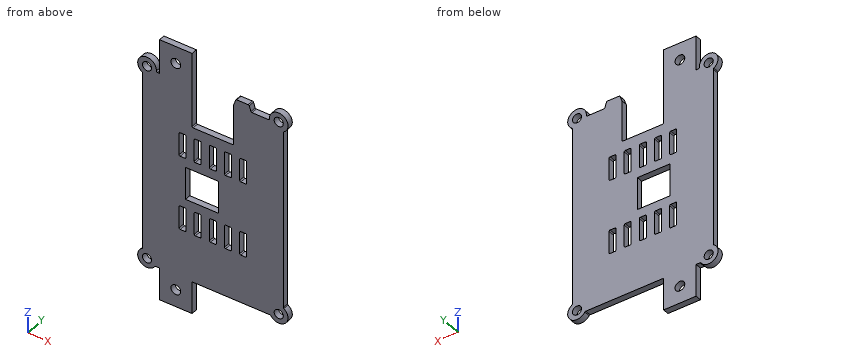
from build123d import *

# Parameters (mm, degrees)
BASEPLATE_OUTLINE_R = 2.1
BASEPLATE_DEPTH     = 2.8
CUT_EXTRUDE1_REACH  = 115.438
SKETCH3_W           = 19.2
SKETCH3_H           = 19.147905432
SKETCH3_W_2         = 15.1
SKETCH3_H_2         = 15.1
SKETCH3_W_3         = 3.2
SKETCH3_H_3         = 11.1
FILLET1_R           = 0.5
SKETCH4_W           = 15
SKETCH4_H           = 35
SKETCH4_R           = 2.25
SKETCH4_H_2         = 15
BOSS_EXTRUDE1_DEPTH = 2.8


# Read off the part's stored shape, not the designer's step: BasePlate
with BuildPart() as part:
    # BasePlate outline → BasePlate (new body)
    with BuildSketch(Plane(origin=(0, 0, 0), x_dir=(1, 0, 0), z_dir=(0, 1, 0))):
        with BuildLine():
            Line((43.502626614, -5.852332608), (48.792614178, -5.852332608))
            ThreePointArc((48.792614178, -5.852332608), (49.082078508, -5.760021707), (49.264659986, -5.517174213))
            Line((49.264659986, -5.517174213), (50.078201202, -3.187491002))
            ThreePointArc((50.078201202, -3.187491002), (50.26078268, -2.944643509), (50.55024701, -2.852332608))
            Line((50.55024701, -2.852332608), (58.116695703, -2.852332608))
            ThreePointArc((58.116695703, -2.852332608), (58.484685739, -3.013831008), (58.614956567, -3.393999275))
            ThreePointArc((58.614956567, -3.393999275), (64.799237397, -7.61016844), (65.229166667, -0.137781095))
            ThreePointArc((65.229166667, -0.137781095), (65.061014427, 0.043158816), (65, 0.282515593))
            Line((65, 0.282515593), (65, 83.012819192))
            ThreePointArc((65, 83.012819192), (65.061014427, 83.252175969), (65.229166667, 83.433115879))
            ThreePointArc((65.229166667, 83.433115879), (65.940559159, 90.088226551), (59.285448487, 89.376834059))
            ThreePointArc((59.285448487, 89.376834059), (59.104508577, 89.208681819), (58.8651518, 89.147667392))
            Line((58.8651518, 89.147667392), (6.1348482, 89.147667392))
            ThreePointArc((6.1348482, 89.147667392), (5.895491423, 89.208681819), (5.714551513, 89.376834059))
            ThreePointArc((5.714551513, 89.376834059), (-0.940559159, 90.088226551), (-0.229166667, 83.433115879))
            ThreePointArc((-0.229166667, 83.433115879), (-0.061014427, 83.252175969), (0, 83.012819192))
            Line((0, 83.012819192), (0, 0.282515593))
            ThreePointArc((0, 0.282515593), (-0.061014427, 0.043158816), (-0.229166667, -0.137781095))
            ThreePointArc((-0.229166667, -0.137781095), (0.200762603, -7.61016844), (6.385043433, -3.393999275))
            ThreePointArc((6.385043433, -3.393999275), (6.515314261, -3.013831008), (6.883304297, -2.852332608))
            Line((6.883304297, -2.852332608), (14.44975299, -2.852332608))
            ThreePointArc((14.44975299, -2.852332608), (14.73921732, -2.944643509), (14.921798798, -3.187491002))
            Line((14.921798798, -3.187491002), (15.735340014, -5.517174213))
            ThreePointArc((15.735340014, -5.517174213), (15.917921492, -5.760021707), (16.207385822, -5.852332608))
            Line((16.207385822, -5.852332608), (21.497373386, -5.852332608))
            ThreePointArc((21.497373386, -5.852332608), (21.786837716, -5.760021707), (21.969419194, -5.517174213))
            Line((21.969419194, -5.517174213), (22.78296041, -3.187491002))
            ThreePointArc((22.78296041, -3.187491002), (22.965541888, -2.944643509), (23.255006218, -2.852332608))
            Line((23.255006218, -2.852332608), (41.744993782, -2.852332608))
            ThreePointArc((41.744993782, -2.852332608), (42.034458112, -2.944643509), (42.21703959, -3.187491002))
            Line((42.21703959, -3.187491002), (43.030580806, -5.517174213))
            ThreePointArc((43.030580806, -5.517174213), (43.213162284, -5.760021707), (43.502626614, -5.852332608))
        make_face()
        with Locations((2.1, -3.752332608)):
            Circle(BASEPLATE_OUTLINE_R, mode=Mode.SUBTRACT)
        with Locations((62.9, -3.752332608)):
            Circle(BASEPLATE_OUTLINE_R, mode=Mode.SUBTRACT)
        with Locations((2.1, 87.047667392)):
            Circle(BASEPLATE_OUTLINE_R, mode=Mode.SUBTRACT)
        with Locations((62.9, 87.047667392)):
            Circle(BASEPLATE_OUTLINE_R, mode=Mode.SUBTRACT)
    extrude(amount=BASEPLATE_DEPTH)

    # Sketch3 → Cut-Extrude1 (cut, up to next)
    with BuildSketch(Plane(origin=(0, 2.8, 0), x_dir=(1, 0, 0), z_dir=(0, 1, 0)), mode=Mode.PRIVATE) as cut_extrude1_sk1:
        with Locations((32.5, 6.573714676)):
            Rectangle(SKETCH3_W, SKETCH3_H)
    cut_extrude1_tool1 = extrude(cut_extrude1_sk1.sketch, amount=-CUT_EXTRUDE1_REACH, mode=Mode.PRIVATE) & part.part
    # Sketch3 → Cut-Extrude1 (cut, up to next)
    with BuildSketch(Plane(origin=(0, 2.8, 0), x_dir=(1, 0, 0), z_dir=(0, 1, 0)), mode=Mode.PRIVATE) as cut_extrude1_sk2:
        with Locations((27.45, 43.897667392)):
            Rectangle(SKETCH3_W_2, SKETCH3_H_2)
    cut_extrude1_tool2 = extrude(cut_extrude1_sk2.sketch, amount=-CUT_EXTRUDE1_REACH, mode=Mode.PRIVATE) & part.part
    # Sketch3 → Cut-Extrude1 (cut, up to next)
    with BuildSketch(Plane(origin=(0, 2.8, 0), x_dir=(1, 0, 0), z_dir=(0, 1, 0)), mode=Mode.PRIVATE) as cut_extrude1_sk3:
        with Locations((32.5, 26.597667392)):
            Rectangle(SKETCH3_W_3, SKETCH3_H_3)
    cut_extrude1_tool3 = extrude(cut_extrude1_sk3.sketch, amount=-CUT_EXTRUDE1_REACH, mode=Mode.PRIVATE) & part.part
    # Sketch3 → Cut-Extrude1 (cut, up to next)
    with BuildSketch(Plane(origin=(0, 2.8, 0), x_dir=(1, 0, 0), z_dir=(0, 1, 0)), mode=Mode.PRIVATE) as cut_extrude1_sk4:
        with Locations((18.5, 26.597667392)):
            Rectangle(SKETCH3_W_3, SKETCH3_H_3)
    cut_extrude1_tool4 = extrude(cut_extrude1_sk4.sketch, amount=-CUT_EXTRUDE1_REACH, mode=Mode.PRIVATE) & part.part
    # Sketch3 → Cut-Extrude1 (cut, up to next)
    with BuildSketch(Plane(origin=(0, 2.8, 0), x_dir=(1, 0, 0), z_dir=(0, 1, 0)), mode=Mode.PRIVATE) as cut_extrude1_sk5:
        with Locations((39.5, 26.597667392)):
            Rectangle(SKETCH3_W_3, SKETCH3_H_3)
    cut_extrude1_tool5 = extrude(cut_extrude1_sk5.sketch, amount=-CUT_EXTRUDE1_REACH, mode=Mode.PRIVATE) & part.part
    # Sketch3 → Cut-Extrude1 (cut, up to next)
    with BuildSketch(Plane(origin=(0, 2.8, 0), x_dir=(1, 0, 0), z_dir=(0, 1, 0)), mode=Mode.PRIVATE) as cut_extrude1_sk6:
        with Locations((46.5, 26.597667392)):
            Rectangle(SKETCH3_W_3, SKETCH3_H_3)
    cut_extrude1_tool6 = extrude(cut_extrude1_sk6.sketch, amount=-CUT_EXTRUDE1_REACH, mode=Mode.PRIVATE) & part.part
    # Sketch3 → Cut-Extrude1 (cut, up to next)
    with BuildSketch(Plane(origin=(0, 2.8, 0), x_dir=(1, 0, 0), z_dir=(0, 1, 0)), mode=Mode.PRIVATE) as cut_extrude1_sk7:
        with Locations((25.5, 26.597667392)):
            Rectangle(SKETCH3_W_3, SKETCH3_H_3)
    cut_extrude1_tool7 = extrude(cut_extrude1_sk7.sketch, amount=-CUT_EXTRUDE1_REACH, mode=Mode.PRIVATE) & part.part
    # Sketch3 → Cut-Extrude1 (cut, up to next)
    with BuildSketch(Plane(origin=(0, 2.8, 0), x_dir=(1, 0, 0), z_dir=(0, 1, 0)), mode=Mode.PRIVATE) as cut_extrude1_sk8:
        with Locations((18.5, 61.197667392)):
            Rectangle(SKETCH3_W_3, SKETCH3_H_3)
    cut_extrude1_tool8 = extrude(cut_extrude1_sk8.sketch, amount=-CUT_EXTRUDE1_REACH, mode=Mode.PRIVATE) & part.part
    # Sketch3 → Cut-Extrude1 (cut, up to next)
    with BuildSketch(Plane(origin=(0, 2.8, 0), x_dir=(1, 0, 0), z_dir=(0, 1, 0)), mode=Mode.PRIVATE) as cut_extrude1_sk9:
        with Locations((32.5, 61.197667392)):
            Rectangle(SKETCH3_W_3, SKETCH3_H_3)
    cut_extrude1_tool9 = extrude(cut_extrude1_sk9.sketch, amount=-CUT_EXTRUDE1_REACH, mode=Mode.PRIVATE) & part.part
    # Sketch3 → Cut-Extrude1 (cut, up to next)
    with BuildSketch(Plane(origin=(0, 2.8, 0), x_dir=(1, 0, 0), z_dir=(0, 1, 0)), mode=Mode.PRIVATE) as cut_extrude1_sk10:
        with Locations((39.5, 61.197667392)):
            Rectangle(SKETCH3_W_3, SKETCH3_H_3)
    cut_extrude1_tool10 = extrude(cut_extrude1_sk10.sketch, amount=-CUT_EXTRUDE1_REACH, mode=Mode.PRIVATE) & part.part
    # Sketch3 → Cut-Extrude1 (cut, up to next)
    with BuildSketch(Plane(origin=(0, 2.8, 0), x_dir=(1, 0, 0), z_dir=(0, 1, 0)), mode=Mode.PRIVATE) as cut_extrude1_sk11:
        with Locations((46.5, 61.197667392)):
            Rectangle(SKETCH3_W_3, SKETCH3_H_3)
    cut_extrude1_tool11 = extrude(cut_extrude1_sk11.sketch, amount=-CUT_EXTRUDE1_REACH, mode=Mode.PRIVATE) & part.part
    # Sketch3 → Cut-Extrude1 (cut, up to next)
    with BuildSketch(Plane(origin=(0, 2.8, 0), x_dir=(1, 0, 0), z_dir=(0, 1, 0)), mode=Mode.PRIVATE) as cut_extrude1_sk12:
        with Locations((25.5, 61.197667392)):
            Rectangle(SKETCH3_W_3, SKETCH3_H_3)
    cut_extrude1_tool12 = extrude(cut_extrude1_sk12.sketch, amount=-CUT_EXTRUDE1_REACH, mode=Mode.PRIVATE) & part.part
    add(cut_extrude1_tool1.solids().sort_by_distance((32.5, 2.8, -6.573715))[0], mode=Mode.SUBTRACT)
    add(cut_extrude1_tool2.solids().sort_by_distance((27.45, 2.8, -43.897667))[0], mode=Mode.SUBTRACT)
    add(cut_extrude1_tool3.solids().sort_by_distance((32.5, 2.8, -26.597667))[0], mode=Mode.SUBTRACT)
    add(cut_extrude1_tool4.solids().sort_by_distance((18.5, 2.8, -26.597667))[0], mode=Mode.SUBTRACT)
    add(cut_extrude1_tool5.solids().sort_by_distance((39.5, 2.8, -26.597667))[0], mode=Mode.SUBTRACT)
    add(cut_extrude1_tool6.solids().sort_by_distance((46.5, 2.8, -26.597667))[0], mode=Mode.SUBTRACT)
    add(cut_extrude1_tool7.solids().sort_by_distance((25.5, 2.8, -26.597667))[0], mode=Mode.SUBTRACT)
    add(cut_extrude1_tool8.solids().sort_by_distance((18.5, 2.8, -61.197667))[0], mode=Mode.SUBTRACT)
    add(cut_extrude1_tool9.solids().sort_by_distance((32.5, 2.8, -61.197667))[0], mode=Mode.SUBTRACT)
    add(cut_extrude1_tool10.solids().sort_by_distance((39.5, 2.8, -61.197667))[0], mode=Mode.SUBTRACT)
    add(cut_extrude1_tool11.solids().sort_by_distance((46.5, 2.8, -61.197667))[0], mode=Mode.SUBTRACT)
    add(cut_extrude1_tool12.solids().sort_by_distance((25.5, 2.8, -61.197667))[0], mode=Mode.SUBTRACT)

    # Fillet1
    fillet1_edges = [part.edges().sort_by_distance(p)[0] for p in [
        (22.9, 1.4, -16.147667392),
        (42.1, 1.4, -16.147667392),
        (37.9, 1.4, -55.647667392),
        (37.9, 1.4, -66.747667392),
        (41.1, 1.4, -66.747667392),
        (41.1, 1.4, -55.647667392),
        (16.9, 1.4, -66.747667392),
        (20.1, 1.4, -66.747667392),
        (20.1, 1.4, -55.647667392),
        (16.9, 1.4, -55.647667392),
        (27.1, 1.4, -66.747667392),
        (27.1, 1.4, -55.647667392),
        (23.9, 1.4, -55.647667392),
        (23.9, 1.4, -66.747667392),
        (30.9, 1.4, -21.047667392),
        (30.9, 1.4, -32.147667392),
        (34.1, 1.4, -32.147667392),
        (34.1, 1.4, -21.047667392),
        (44.9, 1.4, -21.047667392),
        (44.9, 1.4, -32.147667392),
        (48.1, 1.4, -32.147667392),
        (48.1, 1.4, -21.047667392),
        (37.9, 1.4, -21.047667392),
        (37.9, 1.4, -32.147667392),
        (41.1, 1.4, -32.147667392),
        (41.1, 1.4, -21.047667392),
        (16.9, 1.4, -32.147667392),
        (20.1, 1.4, -32.147667392),
        (20.1, 1.4, -21.047667392),
        (16.9, 1.4, -21.047667392),
        (27.1, 1.4, -32.147667392),
        (27.1, 1.4, -21.047667392),
        (23.9, 1.4, -21.047667392),
        (23.9, 1.4, -32.147667392),
        (30.9, 1.4, -55.647667392),
        (30.9, 1.4, -66.747667392),
        (34.1, 1.4, -66.747667392),
        (34.1, 1.4, -55.647667392),
        (44.9, 1.4, -55.647667392),
        (44.9, 1.4, -66.747667392),
        (48.1, 1.4, -66.747667392),
        (48.1, 1.4, -55.647667392),
    ]]
    fillet(fillet1_edges, radius=FILLET1_R)

    # Sketch4 → Boss-Extrude1 (add)
    # profile 1 of 2: a face of its own
    with BuildSketch(Plane(origin=(0, 2.8, 0), x_dir=(1, 0, 0), z_dir=(0, 1, 0))):
        with Locations((15.4, -1.352332608)):
            Rectangle(SKETCH4_W, SKETCH4_H)
        with Locations(Location((15.4, -10.852332608, 0), (0, 0, 270))):
            Circle(SKETCH4_R, mode=Mode.SUBTRACT)
    # profile 2 of 2: a face of its own
    with BuildSketch(Plane(origin=(0, 2.8, 0), x_dir=(1, 0, 0), z_dir=(0, 1, 0))):
        with Locations((15.4, 96.647667392)):
            Rectangle(SKETCH4_W, SKETCH4_H_2)
        with Locations(Location((15.4, 96.147667392, 0), (0, 0, 270))):
            Circle(SKETCH4_R, mode=Mode.SUBTRACT)
    extrude(amount=-BOSS_EXTRUDE1_DEPTH)


solid = part.part
Model file for the job. Use its own axes, mm. Round coordinates to 2 decimals unless told otherwise and drop trailing zeros. Order: outer loops, then holes, each group sorted by start corner. A loop starts at its lowest first (then second) coordinate and runs counter-clockwise, first axis right, second up. Notation, with made-up numbers: M 75,70 L 96,70 A15 cw 96,89 Z; hole C 76,60.25 d4. An arc over 180 degrees is marked long. Write each question's results on one line, items separated by ' | '. Start each with the question number.
(1) Probe probe 1 along Z at (x, y) = (62.9, 1.8); probe 2 along X at (y, z) = (0.7, -58.5); probe 3 along Z at (x, y) = (25, 1.7). List the from-to ranges inside material, lowest first. Write a range as from..to.
(2) Saw through at B-B, the plane x = 2.1. Give the cut face in (y, z).
(3) Saw through at C-C, the plane z = -64. Give the cut face in (x, y), then the cut area to 3 significant figures.
(4) Drop flat-ended pins along their axis: pin 1 (0.7 mm diameter, centred on x = 25.5, y = 1, fed in from +Z); pin 2 (1.4 mm diameter, centred on x = 54.5, y = 1, fed in from +Z); pin 3 (1.4 mm diameter, centred on y = 2, z = -25, fed in from +X). Give the stop position or say it passes through.
(5) Saw through at D-D, the plane x = 15.4. Give the cut face in (y, z).
(6) Saw through at A-A, the plane z = -9.5. Give the cut face in (x, y).
Established:
1) probe 1: z = -91.35..-89.15, -84.95..1.65, 5.85..8.05 | probe 2: x = 0..16.9, 20.1..23.9, 27.1..30.9, 34.1..37.9, 41.1..44.9, 48.1..65 | probe 3: z = -89.15..-66.75, -55.65..-51.45, -36.35..-32.15, -21.05..-16.15
2) outline: M 0,-91.35 L 2.8,-91.35 L 2.8,-89.15 L 0,-89.15 Z; M 0,-84.95 L 2.8,-84.95 L 2.8,1.65 L 0,1.65 Z; M 0,5.85 L 2.8,5.85 L 2.8,8.05 L 0,8.05 Z
3) outline: M 0,0 L 16.9,0 L 16.9,2.8 L 0,2.8 Z; M 20.1,0 L 23.9,0 L 23.9,2.8 L 20.1,2.8 Z; M 27.1,0 L 30.9,0 L 30.9,2.8 L 27.1,2.8 Z; M 34.1,0 L 37.9,0 L 37.9,2.8 L 34.1,2.8 Z; M 41.1,0 L 44.9,0 L 44.9,2.8 L 41.1,2.8 Z; M 48.1,0 L 65,0 L 65,2.8 L 48.1,2.8 Z | area: 137 mm^2
4) pin 1: stops at z = -16.15 | pin 2: stops at z = 2.85 | pin 3: stops at x = 65
5) outline: M 0,-104.15 L 2.8,-104.15 L 2.8,-98.4 L 0,-98.4 Z; M 0,-93.9 L 2.8,-93.9 L 2.8,8.6 L 0,8.6 Z; M 0,13.1 L 2.8,13.1 L 2.8,18.85 L 0,18.85 Z
6) outline: M 0,0 L 22.9,0 L 22.9,2.8 L 0,2.8 Z; M 42.1,0 L 65,0 L 65,2.8 L 42.1,2.8 Z
